Source: CAD feature listing. Evaluate the final solid. Frame: model axes, mm. Face numbers are marked on the shaded views. Give positions to 0.01 mm unless a question says otherwise; leave off trailing zeros. Order: outer loops, then holes, each group sorted by start corner. A loop starts at its lowest first (then second) coordinate and runs counter-clockwise, first axis right, second up. Notation, with made-up numbers: M -14,18 L 13,18 A15 cw 13,47 Z; hole C -39.75,4.5 d6. An arc over 180 degrees is marked long. Use CSV: the item, a comma, the result in double quotes. Start each with the question number.
Item 1: Pull-direction query (X, two-part tool) for the marked faces 1 and 2; classes: +X half, -X half, draft (parallel to the pull), parting line (faces both ways), or undercut.
Item 2: Section query B-B on y = 136.5. Return loops of the section in (x, z).
Item 3: First-contact query: pin 1 (15 mm diameter, centred on x = 747.5, z = 378, fed in from +Y); pin 2 (20.5 mm diameter, centred on y = -131, z = 249.5, fed in from -X); pin 3 (1 mm diameter, centred on x = 178.5, y = -182, fed in from +Z); pin 4 (1 mm diameter, centred on x = 118, y = 47.5, fed in from -Z). Flat tips, straight axial feed; report the tip coordinate or a pass-through.
Item 4: Ray query, probe 1 along Z at (x, y) = (761, -229.5); probe 2 along X at (y, z) = (-173.5, 362); probe 3 along Y at (x, z) = (-398.5, 178.5). Return the intervals inside material, ascending. Write a range as from..to.
Item 5: Section query C-C on z = 560.5. Return loops of the section in (x, y).
Item 6: Section query A-A on z = 88. Return loops of the section in (x, y).
Item 7: Section query D-D on x = -182.5. Return loops of the section in (y, z).
from build123d import *

# Parameters (mm, degrees)
F0_W      = 1346.2
F0_H      = 679.45
F1_DEPTH  = 25.4
F3_W      = 50.8
F3_H      = 317.5
F4_W      = 50.8
F4_H      = 317.5
F5_DEPTH  = 38.1
F7_W      = 50.8
F7_H      = 76.2
F6_W      = 50.8
F6_H      = 76.2
F8_DEPTH  = 660.4
F10_W     = 50.8
F10_H     = 508
F9_W      = 50.8
F9_H      = 508
F11_DEPTH = 25.4
F12_R     = 25.39999
F13_R     = 25.4
F14_W     = 1143.3658423165
F14_H     = 25.4
F15_DEPTH = 304.8


# Not quite as in the source:
# - a fillet or chamfer is up to 0.001 mm smaller than in the source, because OpenCascade refuses the exact size


with BuildPart() as f1:
    # F0 (on Top) → F1 (new body)
    with BuildSketch(Plane.XY):
        with Locations((149.0168645364, 3.430750221)):
            Rectangle(F0_W, F0_H)
    extrude(amount=F1_DEPTH)

    # F3 (on face) + F4 (on face) → F5 (join)
    with BuildSketch(Plane.XY.offset(25.4)):
        with Locations((-433.5340384189, 44.705750221)):
            Rectangle(F3_W, F3_H)
    with BuildSketch(Plane.XY.offset(25.4)):
        with Locations((758.8858046625, 44.705750221)):
            Rectangle(F4_W, F4_H)
    extrude(amount=F5_DEPTH)

    # F7 (on face) + F6 (on face) → F8 (join)
    with BuildSketch(Plane.XY.offset(25.4)):
        with Locations((-433.9627325535, -152.2812862285)):
            Rectangle(F7_W, F7_H)
    with BuildSketch(Plane.XY.offset(25.4)):
        with Locations((758.9168250561, -152.9612190686)):
            Rectangle(F6_W, F6_H)
    extrude(amount=F8_DEPTH)

    # F10 (on face) + F9 (on face) → F11 (join)
    with BuildSketch(Plane.XY.offset(685.8)):
        with Locations((758.9168250561, 14.9119266272)):
            Rectangle(F10_W, F10_H)
    with BuildSketch(Plane.XY.offset(685.8)):
        with Locations((-433.9627325535, 6.5043487549)):
            Rectangle(F9_W, F9_H)
    extrude(amount=F11_DEPTH)

    # F12 (radius 25.4 in the source; OpenCascade refuses exactly that, so slightly less here)
    f12_edges = [f1.edges().sort_by_distance(p)[0] for p in [
        (-459.362733, 260.504349, 698.5),
        (-408.562733, 260.504349, 698.5),
        (733.516825, 268.911927, 698.5),
        (784.316825, 268.911927, 698.5),
        (-459.362733, -247.495651, 698.5),
        (-408.562733, -247.495651, 698.5),
        (733.516825, -239.088073, 698.5),
    ]]
    fillet(f12_edges, radius=F12_R)

    # F13
    f13_edges = [f1.edges().sort_by_distance(p)[0] for p in [
        (784.316825, -239.088073, 698.5),
    ]]
    fillet(f13_edges, radius=F13_R)

    # F14 (on face) → F15 (join)
    with BuildSketch(Plane.XY.offset(25.4)):
        with Locations((163.3197753559, -135.036409986)):
            Rectangle(F14_W, F14_H)
    extrude(amount=F15_DEPTH)


solid = f1.part
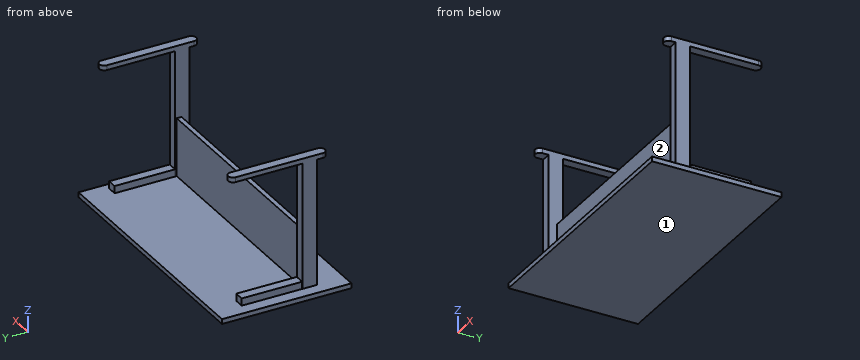
Verdict:
1,face 1,"draft"
1,face 2,"undercut"
2,outline,"M -524.08,0 L 822.12,0 L 822.12,25.4 L 784.29,25.4 L 784.29,63.5 L 733.49,63.5 L 733.49,25.4 L -408.13,25.4 L -408.13,63.5 L -458.93,63.5 L -458.93,25.4 L -524.08,25.4 Z; M -459.36,685.8 L -408.56,685.8 L -408.56,711.2 L -459.36,711.2 Z; M 733.52,685.8 L 784.32,685.8 L 784.32,711.2 L 733.52,711.2 Z"
3,pin 1,"y = -114.86"
3,pin 2,"x = -459.36"
3,pin 3,"z = 25.4"
3,pin 4,"z = 0"
4,probe 1,"0..25.4, 685.8..711.2"
4,probe 2,"-459.36..-408.56, 733.52..784.32"
4,probe 3,"-147.74..-122.34"
5,outline,"M -459.36,-190.38 L -408.56,-190.38 L -408.56,-114.18 L -459.36,-114.18 Z; M 733.52,-191.06 L 784.32,-191.06 L 784.32,-114.86 L 733.52,-114.86 Z"
6,outline,"M -459.36,-190.38 L -408.56,-190.38 L -408.56,-114.18 L -459.36,-114.18 Z; M -408.36,-147.74 L 733.52,-147.74 L 733.52,-191.06 L 784.32,-191.06 L 784.32,-114.86 L 733.52,-114.86 L 733.52,-122.34 L -408.36,-122.34 Z"
7,outline,"M -336.29,0 L 343.16,0 L 343.16,25.4 L -122.34,25.4 L -122.34,330.2 L -147.74,330.2 L -147.74,25.4 L -336.29,25.4 Z"
